Can you work these out from the model? Positions are in its coordinate system, mm. A direction names the side the tool comes from. Give positions to 0.01 mm unless a question says otherwise; leave off trailing zeros. Write each loop counter-clockwise with the first axis right and the second up, starting at its lowest first coordinate (ties: lowest second). Pieces come first, ordered by that corner, then holes. Notation, with made-up numbers: (-37, -10) -> (-19, -10) arc R16 ccw to (-19, 11) -> close; hole circle Ø8 at (66.5, 53.5). An arc over 180 degrees is marked (long way). One line per item, written item: value.
from build123d import *

# Parameters (mm, degrees)
PAD_DEPTH       = 55
SKETCH001_W     = 39
SKETCH001_H     = 45
POCKET_DEPTH    = 54
SKETCH002_R     = 11
SKETCH002_R_2   = 1.6
POCKET001_DEPTH = 45.001
POCKET002_DEPTH = 6.001
FILLET_R        = 2
SKETCH004_W     = 0.885
SKETCH004_H     = 58.852348
POCKET003_DEPTH = 45.001


with BuildPart() as part:
    # Sketch → Pad (new body)
    with BuildSketch(Plane.XY):
        Polygon((0, 0), (0, 60), (6, 60), (45, 6), (45, 0), align=None)
    extrude(amount=PAD_DEPTH)

    # Sketch001 (on Face2 of Pad) → Pocket (cut)
    with BuildSketch(Plane(origin=(0, 60, 0), x_dir=(-1, 0, 0), z_dir=(0, 1, 0))):
        with Locations((-25.5, 27.5)):
            Rectangle(SKETCH001_W, SKETCH001_H)
    extrude(amount=-POCKET_DEPTH, mode=Mode.SUBTRACT)

    # Sketch002 (on Face1 of Pocket) → Pocket001 (cut, through all)
    with BuildSketch(Plane(origin=(0, 0, 0), x_dir=(0, -1, 0), z_dir=(-1, 0, 0))):
        with Locations((-39.2, 27.5)):
            Circle(SKETCH002_R)
        with Locations((-54.2, 27.5)):
            Circle(SKETCH002_R_2)
        with Locations((-31.7, 40.4904)):
            Circle(SKETCH002_R_2)
        with Locations((-31.7, 14.5096)):
            Circle(SKETCH002_R_2)
    extrude(amount=-POCKET001_DEPTH, mode=Mode.SUBTRACT)

    # Sketch003 (on Face14 of Pocket001) → Pocket002 (cut, through all)
    with BuildSketch(Plane(origin=(0, 6, 0), x_dir=(-1, 0, 0), z_dir=(0, 1, 0))):
        with BuildLine():
            ThreePointArc((-35.5, 40.1), (-38.1, 37.5), (-35.5, 34.9))
            Line((-35.5, 34.9), (-15.5, 34.9))
            ThreePointArc((-15.5, 34.9), (-12.9, 37.5), (-15.5, 40.1))
            Line((-15.5, 40.1), (-35.5, 40.1))
        make_face()
        with BuildLine():
            ThreePointArc((-35.5, 20.1), (-38.1, 17.5), (-35.5, 14.9))
            Line((-35.5, 14.9), (-15.5, 14.9))
            ThreePointArc((-15.5, 14.9), (-12.9, 17.5), (-15.5, 20.1))
            Line((-15.5, 20.1), (-35.5, 20.1))
        make_face()
    extrude(amount=-POCKET002_DEPTH, mode=Mode.SUBTRACT)

    # Fillet
    fillet_edges = [part.edges().sort_by_distance(p)[0] for p in [
        (3, 60, 55),
        (3, 60, 0),
        (45, 3, 0),
        (45, 3, 55),
    ]]
    fillet(fillet_edges, radius=FILLET_R)

    # Sketch004 (on Face14 of Fillet) → Pocket003 (cut, through all)
    with BuildSketch(Plane.YZ.offset(45)):
        with Locations((0.4425, 29.426174)):
            Rectangle(SKETCH004_W, SKETCH004_H)
    extrude(amount=-POCKET003_DEPTH, mode=Mode.SUBTRACT)


solid = part.part
1) If we section it at A-A (z = 27.5): Write out the boundary of the cut face in (x, y) (3 decimals), and give its area (3 significant figures).
Answer list:
outline: (0, 0.885) -> (45, 0.885) -> (45, 6) -> (6, 6) -> (6, 28.2) -> (0, 28.2) -> close; (0, 50.2) -> (6, 50.2) -> (6, 52.6) -> (0, 52.6) -> close; (0, 55.8) -> (6, 55.8) -> (6, 60) -> (0, 60) -> close
area: 403 mm^2
2) If we section it at D-D (y = 15.5): Write out the boundary of the cut face in (x, z), and give its area (3 significant figures).
Answer list:
outline: (0, 0) -> (38.14, 0) -> (38.14, 5) -> (6, 5) -> (6, 50) -> (38.14, 50) -> (38.14, 55) -> (0, 55) -> close
area: 651 mm^2
3) If we section it at B-B (x = 25): Write out the boundary of the cut face in (y, z) (3 decimals), and give its area (3 significant figures).
Answer list:
outline: (0.885, 0) -> (33.692, 0) -> (33.692, 5) -> (6, 5) -> (6, 14.9) -> (0.885, 14.9) -> close; (0.885, 20.1) -> (6, 20.1) -> (6, 34.9) -> (0.885, 34.9) -> close; (0.885, 40.1) -> (6, 40.1) -> (6, 50) -> (33.692, 50) -> (33.692, 55) -> (0.885, 55) -> close
area: 505 mm^2
4) If we section it at C-C (y = 35): Write out the boundary of the cut face in (x, z), and give its area (3 significant figures).
Answer list:
outline: (0, 0) -> (24.06, 0) -> (24.06, 5) -> (6, 5) -> (6, 17.33) -> (0, 17.33) -> close; (0, 37.67) -> (6, 37.67) -> (6, 50) -> (24.06, 50) -> (24.06, 55) -> (0, 55) -> close
area: 389 mm^2
5) I need wall thicknesses on L1, parallel to Z at x = 3.1, y = 39.2; L2, parallel to Z at x = 1, y = 54; L3, parallel to Z at x = 4, y = 31. Which ranges of each line are inside material? Lowest first, please.
Answer list:
L1: z = 0 to 16.5, 38.5 to 55
L2: z = 0 to 25.91, 29.09 to 55
L3: z = 0 to 13.07, 15.95 to 20.17, 34.83 to 39.05, 41.93 to 55
6) We'd pull the mould along Z, two halves only. Please class faces 4 (the face through (12.9, 3.5, 37.4)), 5 (the face through (45, 3, 27)), 6 (the face through (2.95, 59.4, 54.43)): released by +Z, released by -Z, zero draft, split by the parting line, or undercut.
Answer list:
face 4: undercut
face 5: zero draft
face 6: released by +Z
7) For faces 1 (the face through (26, 6, 28)), 2 (the face through (2.958, 30.174, 40.971)), 3 (the face through (25, 3, 40.1)), which set-ups out of +Z, -Z, +X, -X, +Y, -Y let a thin tool reach every point of the face, with its end or its side?
Answer list:
face 1: +X, +Y
face 2: +X, -X
face 3: +Y, -Y
8) Will these pins go through, and if not, where does the flat tip stop? pin 1 (3.5 mm diameter, centred on y = 31.7, z = 14.51, fed in from +X); pin 2 (3 mm diameter, centred on x = 28, z = 28, fed in from +Y); pin 3 (3 mm diameter, centred on y = 54.2, z = 27.5, fed in from +X).
Answer list:
pin 1: stops at x = 6
pin 2: stops at y = 6
pin 3: passes through
